Geometry: final body of the model. Coordinates: model frame, mm. A direction names the side the tool comes from. Round coordinates to 2 decimals unless told otherwise and drop trailing zeros. Loops run counter-clockwise (first coordinate to the right, second up) from the corner with the lowest first, then second, coordinate; pieces in that order, holes last. Notation, with made-up numbers: (77, -32) - (110, -32) arc R18 ccw to (110, 2) - close; hole circle Ø1 at (-36, 24). An arc over 180 degrees is marked (long way). Return JSON: item names as keys, results as strings. Group by question number.
1. Draft query along X for faces 1 (the face through (22.5, 1, -21)), 2 (the face through (0, -10, -22)), 3 (the face through (-21.6, -11.64, -21.55)). Return one class per face: +X half, -X half, draft (parallel to the pull), parting line (faces both ways), or undercut.
2. Section C-C on y = 0. Return loops of the section in (x, z), and give its area (4 significant figures).
3. First-contact query: pin 1 Ø20 at (x, z) = (0, -13.5) entering from +Y; pin 2 Ø6 at (x, y) = (-2, -6.5) entering from -Z; pin 3 Ø6.5 at (x, z) = (10, -21.1) entering from -Y; pin 4 Ø3.5 at (x, z) = (-10, -21.1) entering from -Y. Flat tips, straight axial feed; report the tip coordinate or a pass-through.
4. Set-up query: faces 4 (the face through (0, -12.5, -21)), 5 (the face through (0, 1, -2.5)). Return all of +Z, -Z, +X, -X, +Y, -Y with unobstructed straight access to the full face (end or side cutting, diameter ignored); none if empty.
5. Material intervals for probe 1 along X at (y, z) = (10.25, -39); probe 2 along X at (y, z) = (-11.15, -21.1); probe 3 along X at (y, z) = (-11.65, -21.1), sorted ascending.
6. Section A-A on x = -10. Return loops of the section in (y, z).
7. Section D-D on z = -13. Return loops of the section in (x, y).
8. Section B-B on z = -21.1. Return loops of the section in (x, y), and give its area (3 significant figures).
from build123d import *

# Parameters (mm, degrees)
CROQUIS1_W              = 45
CROQUIS1_H              = 25
SALIENTE_EXTRUIR1_DEPTH = 2.5
SALIENTE_EXTRUIR2_DEPTH = 40
REDONDEO2_R             = 3
REDONDEO3_R             = 3
CROQUIS3_R              = 2
CORTAR_EXTRUIR1_DEPTH   = 100
CROQUIS4_R              = 2
CORTAR_EXTRUIR2_DEPTH   = 40


with BuildPart() as part:
    # Croquis1 → Saliente-Extruir1 (new body)
    with BuildSketch(Plane.XY):
        Rectangle(CROQUIS1_W, CROQUIS1_H)
    extrude(amount=-SALIENTE_EXTRUIR1_DEPTH)

    # Croquis2 → Saliente-Extruir2 (add)
    with BuildSketch(Plane(origin=(0, 0, -2.5), x_dir=(-1, 0, 0), z_dir=(0, 0, -1))):
        Polygon((-22.5, 12.5), (-20, 12.5), (-20, -10), (20, -10), (20, 12.5), (22.5, 12.5), (22.5, -12.5), (20, -12.5), (-20, -12.5), (-22.5, -12.5), align=None)
    extrude(amount=SALIENTE_EXTRUIR2_DEPTH)

    # Redondeo2
    redondeo2_edges = [part.edges().sort_by_distance(p)[0] for p in [
        (22.5, -12.5, -21.25),
    ]]
    fillet(redondeo2_edges, radius=REDONDEO2_R)

    # Redondeo3
    redondeo3_edges = [part.edges().sort_by_distance(p)[0] for p in [
        (-22.5, -12.5, -21.25),
    ]]
    fillet(redondeo3_edges, radius=REDONDEO3_R)

    # Croquis3 → Cortar-Extruir1 (cut)
    with BuildSketch(Plane(origin=(22.5, 0, 0), x_dir=(0, 0, -1), z_dir=(1, 0, 0))):
        with Locations((10, 0)):
            Circle(CROQUIS3_R)
    extrude(amount=-CORTAR_EXTRUIR1_DEPTH, mode=Mode.SUBTRACT)

    # Croquis4 → Cortar-Extruir2 (cut)
    with BuildSketch(Plane.XZ.offset(12.5)):
        with Locations(Location((-10, -21.1, 0), (0, 0, 270))):
            Circle(CROQUIS4_R)
        with Locations(Location((10, -21.1, 0), (0, 0, 270))):
            Circle(CROQUIS4_R)
    extrude(amount=-CORTAR_EXTRUIR2_DEPTH, mode=Mode.SUBTRACT)


solid = part.part
Taken from the geometry:
{
 "1": {"face 1": "+X half", "face 2": "undercut", "face 3": "-X half"},
 "2": {"outline": "(-22.5, -42.5) - (-20, -42.5) - (-20, -12) - (-22.5, -12) - close; (-22.5, -8) - (-20, -8) - (-20, -2.5) - (20, -2.5) - (20, -8) - (22.5, -8) - (22.5, 0) - (-22.5, 0) - close; (20, -42.5) - (22.5, -42.5) - (22.5, -12) - (20, -12) - close", "area": "292.5 mm2"},
 "3": {"pin 1": "y = -10", "pin 2": "z = -2.5", "pin 3": "y = -12.5", "pin 4": "through"},
 "4": {"face 4": "+Z, -Z, +X, -X, -Y", "face 5": "-Z, +Y"},
 "5": {"probe 1": "-22.5 to -20, 20 to 22.5", "probe 2": "-22.01 to -12, -8 to 8, 12 to 22.01", "probe 3": "-21.59 to -12, -8 to 8, 12 to 21.59"},
 "6": {"outline": "(-12.5, -42.5) - (-10, -42.5) - (-10, -23.1) - (-12.5, -23.1) - close; (-12.5, -19.1) - (-10, -19.1) - (-10, -2.5) - (12.5, -2.5) - (12.5, 0) - (-12.5, 0) - close"},
 "7": {"outline": "(-22.5, -9.5) arc R3 ccw to (-19.5, -12.5) - (19.5, -12.5) arc R3 ccw to (22.5, -9.5) - (22.5, 12.5) - (20, 12.5) - (20, -10) - (-20, -10) - (-20, 12.5) - (-22.5, 12.5) - close"},
 "8": {"outline": "(-22.5, -9.5) arc R3 ccw to (-19.5, -12.5) - (-12, -12.5) - (-12, -10) - (-20, -10) - (-20, 12.5) - (-22.5, 12.5) - close; (-8, -12.5) - (8, -12.5) - (8, -10) - (-8, -10) - close; (12, -12.5) - (19.5, -12.5) arc R3 ccw to (22.5, -9.5) - (22.5, 12.5) - (20, 12.5) - (20, -10) - (12, -10) - close", "area": "201 mm2"}
}
